Autodesk Inventor part; units mm, degrees
ref_plane "YZ Plane" through (0, 0, 0) normal (1, 0, 0) x (0, 1, 0)
ref_plane "XZ Plane" through (0, 0, 0) normal (0, 1, 0) x (-1, 0, 0)
ref_plane "XY Plane" through (0, 0, 0) normal (0, 0, 1) x (1, 0, 0)
sketch "Sketch1" plane through (0, 0, 0) normal (0, 0, 1) x (1, 0, 0)
  line L0 (0, 0) -> (38.1, 0)
  line L1 (38.1, 0) -> (38.1, 38.1)
  line L2 (38.1, 38.1) -> (0, 38.1)
  line L3 (0, 38.1) -> (0, 0)
  dimension "d0" = 38.1
  dimension "d1" = 38.1
extrude "Extrusion1" add sketch "Sketch1" along normal blind 38.1
sketch "Sketch2" plane through (0, 0, 38.1) normal (0, 0, 1) x (1, 0, 0)
  line L0 (6.35, 6.35) -> (32.004, 6.35)
  line L1 (32.004, 6.35) -> (32.004, 32.004)
  line L2 (32.004, 32.004) -> (6.35, 32.004)
  line L3 (6.35, 32.004) -> (6.35, 6.35)
  line L4 (38.1, 0) -> (38.1, 38.1)
  line L5 (0, 0) -> (38.1, 0)
  line L6 (38.1, 0) -> (38.1, 38.1)
  line L7 (38.1, 38.1) -> (0, 38.1)
  line L8 (0, 38.1) -> (0, 0)
  dimension "d4" = 25.654
  dimension "d5" = 25.654
extrude "Extrusion2" cut sketch "Sketch2" against normal blind 31.75 contours L3 L2 L1 L0
sketch "Sketch5" plane through (0, 0, 38.1) normal (0, 0, 1) x (1, 0, 0)
  line L0 (6.35, 6.35) -> (6.35, 32.004)
  line L1 (6.35, 6.35) -> (32.004, 6.35)
  line L2 (32.004, 6.35) -> (32.004, 32.004)
  line L3 (32.004, 32.004) -> (6.35, 32.004)
  line L4 (6.35, 32.004) -> (6.35, 6.35)
  line L5 (0, 0) -> (38.1, 0)
  line L6 (0, 0) -> (38.1, 0)
  line L7 (38.1, 0) -> (38.1, 38.1)
  line L8 (38.1, 38.1) -> (0, 38.1)
  line L9 (0, 38.1) -> (0, 0)
extrude "Extrusion4" add sketch "Sketch5" along normal blind 38.1
sketch "Sketch7" plane through (38.1, 0, 0) normal (1, 0, 0) x (0, 0, -1)
  line L0 (0, 0) -> (-76.2, 0)
  line L1 (0, 0) -> (-38.1, 0)
  line L2 (-38.1, 0) -> (-38.1, 38.1)
  line L3 (-38.1, 38.1) -> (0, 38.1)
  line L4 (0, 38.1) -> (0, 0)
  line L5 (-76.2, 6.35) -> (-6.35, 6.35)
  line L6 (-6.35, 6.35) -> (-32.004, 6.35)
  line L7 (-32.004, 6.35) -> (-32.004, 32.004)
  line L8 (-32.004, 32.004) -> (-6.35, 32.004)
  line L9 (-6.35, 32.004) -> (-6.35, 6.35)
  dimension "d16" = 38.1
  dimension "d17" = 38.1
  dimension "d20" = 25.654
  dimension "d21" = 25.654
extrude "Extrusion6" add sketch "Sketch7" along normal blind 38.1
sketch "Sketch9" plane through (38.1, 6.35, 6.35) normal (1, 0, 0) x (0, 0, -1)
  line L0 (-25.654, 0) -> (-25.654, 25.654)
  line L1 (0, 0) -> (0, 25.654)
  line L2 (-25.654, 0) -> (0, 0)
  line L3 (0, 0) -> (0, 25.654)
  line L4 (0, 25.654) -> (-25.654, 25.654)
  line L5 (-25.654, 25.654) -> (-25.654, 0)
  point P0 (6.35, -6.35)
extrude "Extrusion7" cut sketch "Sketch9" against normal blind 31.75
sketch "Sketch10" plane through (0, 38.1, 76.2) normal (0, 1, 0) x (1, 0, 0)
  line L0 (76.2, 69.85) -> (6.35, 69.85)
  line L1 (6.35, 69.85) -> (32.004, 69.85)
  line L2 (32.004, 69.85) -> (32.004, 44.196)
  line L3 (32.004, 44.196) -> (6.35, 44.196)
  line L4 (6.35, 44.196) -> (6.35, 69.85)
  line L5 (38.1, 38.1) -> (38.1, 0)
  line L6 (0, 76.2) -> (0, 0)
  line L7 (38.1, 38.1) -> (0, 38.1)
  line L8 (0, 38.1) -> (0, 76.2)
  line L9 (0, 76.2) -> (38.1, 76.2)
  line L10 (38.1, 76.2) -> (38.1, 38.1)
  point P0 (0, 38.1)
  dimension "d26" = 25.654
  dimension "d27" = 25.654
extrude "Extrusion8" add sketch "Sketch10" along normal blind 38.1
sketch "Sketch11" plane through (6.35, 38.1, 6.35) normal (0, 1, 0) x (1, 0, 0)
  line L0 (0, -25.654) -> (25.654, -25.654)
  line L1 (25.654, -25.654) -> (0, -25.654)
  line L2 (0, -25.654) -> (0, 0)
  line L3 (0, 0) -> (25.654, 0)
  line L4 (25.654, 0) -> (25.654, -25.654)
  point P0 (-6.35, 6.35)
extrude "Extrusion9" cut sketch "Sketch11" against normal blind 6.35
sketch "Sketch12" plane through (0, 76.2, 76.2) normal (0, 1, 0) x (1, 0, 0)
  line L0 (38.1, 55.88) -> (32.004, 55.88)
  line L1 (32.004, 55.88) -> (32.004, 58.42)
  line L2 (32.004, 58.42) -> (38.1, 58.42)
  line L3 (38.1, 58.42) -> (38.1, 55.88)
  point P0 (0, 76.2)
  dimension "d32" = 6.096
  dimension "d33" = 2.54
extrude "Extrusion10" cut sketch "Sketch12" against normal blind 38.1
sketch "Sketch13" plane through (76.2, 38.1, 38.1) normal (0, 1, 0) x (1, 0, 0)
  line L0 (0, 31.75) -> (0, 6.096)
  line L1 (-44.196, 17.78) -> (0, 17.78)
  line L2 (0, 17.78) -> (0, 20.32)
  line L3 (0, 20.32) -> (-44.196, 20.32)
  line L4 (-44.196, 20.32) -> (-44.196, 17.78)
  point P0 (-76.2, 38.1)
  dimension "d36" = 2.54
extrude "Extrusion11" cut sketch "Sketch13" against normal blind 6.35
sketch "Sketch15" plane through (0, 76.2, 76.2) normal (0, 1, 0) x (1, 0, 0)
  line L0 (17.78, 38.1) -> (20.32, 38.1)
  line L1 (20.32, 38.1) -> (20.32, 44.196)
  line L2 (20.32, 44.196) -> (17.78, 44.196)
  line L3 (17.78, 44.196) -> (17.78, 38.1)
  point P0 (0, 76.2)
  dimension "d39" = 2.54
  dimension "d40" = 6.096
extrude "Extrusion12" cut sketch "Sketch15" against normal blind 38.1
sketch "Sketch16" plane through (0, 38.1, 76.2) normal (0, 1, 0) x (1, 0, 0)
  line L0 (20.32, 44.196) -> (20.32, 38.1)
  line L1 (0, 0) -> (38.1, 0)
  line L2 (20.32, 44.196) -> (17.78, 44.196)
  line L3 (17.78, 44.196) -> (17.78, 0)
  line L4 (17.78, 0) -> (20.32, 0)
  line L5 (20.32, 0) -> (20.32, 44.196)
  point P0 (0, 76.2)
  dimension "d43" = 2.54
extrude "Extrusion13" cut sketch "Sketch16" against normal blind 6.35
sketch "Sketch17" plane through (38.1, 0, 76.2) normal (1, 0, 0) x (0, 0, -1)
  line L0 (38.1, 0) -> (38.1, 38.1)
  line L1 (0, 17.78) -> (38.1, 17.78)
  line L2 (38.1, 17.78) -> (38.1, 20.32)
  line L3 (38.1, 20.32) -> (0, 20.32)
  line L4 (0, 20.32) -> (0, 17.78)
  point P0 (76.2, 0)
  dimension "d46" = 2.54
extrude "Extrusion14" cut sketch "Sketch17" against normal blind 6.35
sketch "Sketch18" plane through (38.1, 0, 38.1) normal (0, 0, 1) x (1, 0, 0)
  line L0 (0, 17.78) -> (38.1, 17.78)
  line L1 (38.1, 17.78) -> (38.1, 20.32)
  line L2 (38.1, 20.32) -> (0, 20.32)
  line L3 (0, 20.32) -> (0, 17.78)
  point P0 (-38.1, 0)
  dimension "d49" = 38.1
  dimension "d50" = 2.54
extrude "Extrusion15" cut sketch "Sketch18" against normal blind 6.35
sketch "Sketch20" plane through (38.1, 38.1, 38.1) normal (0, 0, 1) x (1, 0, 0)
  line L0 (-17.78, -6.096) -> (-17.78, 38.1)
  line L1 (0, 0) -> (-17.78, 0)
  line L2 (-17.78, 38.1) -> (-16.51, 38.1)
  line L3 (-16.51, 38.1) -> (-16.51, 0)
  line L4 (-16.51, 0) -> (-17.78, 0)
  line L5 (-17.78, 0) -> (-17.78, 38.1)
  point P0 (-38.1, -38.1)
  dimension "d53" = 1.27
extrude "Extrusion16" cut sketch "Sketch20" against normal blind 6.35
sketch "Sketch21" plane through (38.1, 38.1, 76.2) normal (0, 1, 0) x (1, 0, 0)
  line L0 (-17.78, 0) -> (-17.78, 44.196)
  line L1 (0, 0) -> (-17.78, 0)
  line L2 (-17.78, 44.196) -> (-16.51, 44.196)
  line L3 (-16.51, 44.196) -> (-16.51, 0)
  line L4 (-16.51, 0) -> (-17.78, 0)
  line L5 (-17.78, 0) -> (-17.78, 44.196)
  point P0 (-38.1, 76.2)
  dimension "d56" = 1.27
extrude "Extrusion17" cut sketch "Sketch21" against normal blind 6.35
sketch "Sketch23" plane through (0, 38.1, 38.1) normal (0, 0, 1) x (1, 0, 0)
  line L0 (17.78, 0) -> (17.78, 38.1)
  line L1 (17.78, 0) -> (0, 0)
  line L2 (17.78, 38.1) -> (16.51, 38.1)
  line L3 (16.51, 38.1) -> (16.51, 0)
  line L4 (16.51, 0) -> (17.78, 0)
  line L5 (17.78, 0) -> (17.78, 38.1)
  point P0 (0, -38.1)
  dimension "d59" = 1.27
extrude "Extrusion18" cut sketch "Sketch23" against normal blind 6.35
sketch "Sketch24" plane through (0, 38.1, 76.2) normal (0, 1, 0) x (1, 0, 0)
  line L0 (17.78, 44.196) -> (17.78, 0)
  line L1 (17.78, 0) -> (0, 0)
  line L2 (17.78, 44.196) -> (16.51, 44.196)
  line L3 (16.51, 44.196) -> (16.51, 0)
  line L4 (16.51, 0) -> (17.78, 0)
  line L5 (17.78, 0) -> (17.78, 44.196)
  point P0 (0, 76.2)
  dimension "d62" = 1.27
extrude "Extrusion19" cut sketch "Sketch24" against normal blind 6.35
sketch "Sketch25" plane through (38.1, 0, 76.2) normal (1, 0, 0) x (0, 0, -1)
  line L0 (38.1, 0) -> (38.1, 17.78)
  line L1 (38.1, 17.78) -> (0, 17.78)
  line L2 (0, 17.78) -> (0, 16.51)
  line L3 (0, 16.51) -> (38.1, 16.51)
  line L4 (38.1, 16.51) -> (38.1, 17.78)
  point P0 (76.2, 0)
  dimension "d65" = 38.1
  dimension "d66" = 1.27
extrude "Extrusion20" cut sketch "Sketch25" against normal blind 6.35
sketch "Sketch26" plane through (38.1, 38.1, 76.2) normal (1, 0, 0) x (0, 0, -1)
  line L0 (0, -17.78) -> (38.1, -17.78)
  line L1 (38.1, -17.78) -> (0, -17.78)
  line L2 (0, -17.78) -> (0, -16.51)
  line L3 (0, -16.51) -> (38.1, -16.51)
  line L4 (38.1, -16.51) -> (38.1, -17.78)
  point P0 (76.2, -38.1)
  dimension "d69" = 38.1
  dimension "d70" = 1.27
extrude "Extrusion21" cut sketch "Sketch26" against normal blind 6.35
sketch "Sketch27" plane through (38.1, 0, 38.1) normal (0, 0, 1) x (1, 0, 0)
  line L0 (0, 21.59) -> (0, 38.1)
  line L1 (0, 20.32) -> (38.1, 20.32)
  line L2 (0, 21.59) -> (38.1, 21.59)
  line L3 (38.1, 21.59) -> (38.1, 20.32)
  line L4 (38.1, 20.32) -> (0, 20.32)
  line L5 (0, 20.32) -> (0, 21.59)
  line L6 (38.1, 17.78) -> (0, 17.78)
  line L7 (0, 17.78) -> (38.1, 17.78)
  line L8 (38.1, 17.78) -> (38.1, 16.51)
  line L9 (38.1, 16.51) -> (0, 16.51)
  line L10 (0, 16.51) -> (0, 17.78)
  point P0 (-38.1, 0)
  dimension "d73" = 38.1
  dimension "d74" = 1.27
extrude "Extrusion22" cut sketch "Sketch27" against normal blind 6.35
sketch "Sketch28" plane through (38.1, 38.1, 38.1) normal (0, 1, 0) x (1, 0, 0)
  line L0 (0, 20.32) -> (38.1, 20.32)
  line L1 (0, 20.32) -> (38.1, 20.32)
  line L2 (38.1, 20.32) -> (38.1, 21.59)
  line L3 (38.1, 21.59) -> (0, 21.59)
  line L4 (0, 21.59) -> (0, 20.32)
  line L5 (-6.096, 17.78) -> (38.1, 17.78)
  line L6 (38.1, 17.78) -> (0, 17.78)
  line L7 (0, 17.78) -> (0, 16.51)
  line L8 (0, 16.51) -> (38.1, 16.51)
  line L9 (38.1, 16.51) -> (38.1, 17.78)
  point P0 (-38.1, 38.1)
  point P1 (0, 17.78)
  dimension "d77" = 38.1
  dimension "d78" = 1.27
  dimension "d79" = 38.1
  dimension "d80" = 1.27
extrude "Extrusion23" cut sketch "Sketch28" against normal blind 6.35
sketch "Sketch29" plane through (38.1, 38.1, 0) normal (1, 0, 0) x (0, 0, -1)
  line L0 (-17.78, -6.096) -> (-6.35, -6.096)
  line L1 (-6.35, 38.1) -> (-17.78, 38.1)
  line L2 (-17.78, -6.096) -> (-16.51, -6.096)
  line L3 (-16.51, -6.096) -> (-16.51, 38.1)
  line L4 (-16.51, 38.1) -> (-17.78, 38.1)
  line L5 (-17.78, 38.1) -> (-17.78, -6.096)
  line L6 (-21.59, 0) -> (-21.59, -6.096)
  line L7 (-20.32, 38.1) -> (-20.32, -6.096)
  line L8 (-21.59, -6.096) -> (-20.32, -6.096)
  line L9 (-20.32, -6.096) -> (-20.32, 38.1)
  line L10 (-20.32, 38.1) -> (-21.59, 38.1)
  line L11 (-21.59, 38.1) -> (-21.59, -6.096)
  point P0 (0, -38.1)
  point P1 (-20.32, -6.096)
  dimension "d83" = 1.27
extrude "Extrusion24" cut sketch "Sketch29" against normal blind 6.35
sketch "Sketch30" plane through (76.2, 38.1, 21.59) normal (0, 0, -1) x (-1, 0, 0)
  line L0 (0, 0) -> (38.1, 0)
  line L1 (44.196, 38.1) -> (44.196, -6.096)
  line L2 (38.1, 0) -> (44.196, 0)
  line L3 (44.196, 0) -> (44.196, -6.096)
  line L4 (44.196, -6.096) -> (38.1, -6.096)
  line L5 (38.1, -6.096) -> (38.1, 0)
  point P0 (76.2, -38.1)
  point P1 (44.196, 0)
extrude "Extrusion25" add sketch "Sketch30" along normal blind 5.08
sketch "Sketch31" plane through (21.59, 38.1, 38.1) normal (-1, 0, 0) x (0, 0, 1)
  line L0 (38.1, -6.096) -> (-6.096, -6.096)
  line L1 (0, 0) -> (-6.096, 0)
  line L2 (-6.096, 0) -> (-6.096, -6.096)
  line L3 (-6.096, -6.096) -> (0, -6.096)
  line L4 (0, -6.096) -> (0, 0)
  point P0 (-38.1, -38.1)
extrude "Extrusion26" add sketch "Sketch31" along normal blind 5.08
sketch "Sketch32" plane through (0, 0, 76.2) normal (-1, 0, 0) x (0, 0, 1)
  line L0 (0, 38.1) -> (0, 0)
  line L1 (0, 19.05) -> (-76.2, 19.05)
  line L2 (-76.2, 19.05) -> (-76.2, 0)
  line L3 (-76.2, 0) -> (0, 0)
  line L4 (0, 0) -> (0, 19.05)
  line L5 (-76.2, 0) -> (-56.896, 0)
  line L6 (-56.896, 0) -> (-56.896, 76.2)
  line L7 (-56.896, 76.2) -> (-76.2, 76.2)
  line L8 (-76.2, 76.2) -> (-76.2, 0)
  point P0 (0, 0)
  point P1 (-56.896, 19.05)
  dimension "d90" = 19.304
  dimension "d91" = 76.2
extrude "Extrusion27" add sketch "Sketch32" along normal blind 12.7 contours L6 L3 L2 L1 | L1 L8 L7 L6
sketch "Sketch35" plane through (-12.7, 0, 76.2) normal (-1, 0, 0) x (0, 0, 1)
  line L0 (-38.1, 38.1) -> (-38.1, 76.2)
  line L1 (-38.1, 76.2) -> (-56.896, 76.2)
  line L2 (-56.896, 76.2) -> (-56.896, 0)
  line L3 (-56.896, 0) -> (-38.1, 0)
  line L4 (-38.1, 0) -> (-38.1, 76.2)
  point P0 (-76.2, 0)
  dimension "d102" = 18.796
  dimension "d103" = 76.2
extrude "Extrusion30" add sketch "Sketch35" against normal blind 6.35
properties part number "corner connector with rails (front left)"
Build history of the part. All positions in model axes, mm. A direction names the side the tool comes from. Coordinates: 2 decimals unless noted, no trailing zeros. Write each loop counter-clockwise with the first axis right and the second up, starting at its lowest first coordinate (ties: lowest second). Pieces come first, ordered by that corner, then holes. Notation, with made-up numbers: (-21, 49.5) -> (38, 49.5) arc R27 ccw to (38, 80.5) -> close; hole circle Ø8 at (20, 9.25). An arc over 180 degrees is marked (long way). Use CSV: the item, a comma, the result in double quotes. Start each with the question number.
Q1. Cut at A-A, the plane z = 23.5. List the corners of the cut face in (x, y), then the cut area to 3 significant figures.
Q2. Cut at C-C, the plane y = 23. List the corners of the cut face in (x, z).
Q3. 3-axis set-ups, long thin cutter, end or side, ignore diameter. For faces 1 (the flat face through (57, 30, 38.1)), 2 (the flat face through (21.59, 57, 35)), 3 (the flat face through (57, 35, 21.59)): which of +Z, -Z, +X, -X, +Y, -Y reach the whole face in a straight line?
Q4. Cut at D-D, the plane z = 61. List the corners of the cut face in (x, y).
Q5. Pull direction Z, two halves, no side cores. Call faces 4 (the flat face through (-6.35, 39, 29)), 5 (the flat face through (38.1, 35, 19)), 6 (the flat face through (-3, 38, 19.304)): released by +Z, released by -Z, zero draft, split by the parting line, or undercut.
Q6. Cut at B-B, the plane x = 11.5. List the corners of the cut face in (y, z), then the cut area to 3 significant figures.
Q7. Drill centre lines: probe 1 along X at (y, z) = (59.5, 30.5); probe 2 along X at (y, z) = (37.5, 70.5); probe 3 along Z at (x, y) = (44, 25.5). Where is each one in solid material? Low to high.
Q8. Flat gauge pins, fed straight in: pin 1 Ø6.5 at (x, y) = (57, 36.5) entering from +Z; pin 2 Ø1.5 at (x, z) = (1, 52.5) entering from +Y; pin 3 Ø5 at (y, z) = (19.5, 48) entering from -X. Where does each tip first touch, or does it go through?
Checked values:
1,outline,"(-12.7, 0) -> (-6.35, 0) -> (-6.35, 76.2) -> (-12.7, 76.2) -> close; (0, 0) -> (76.2, 0) -> (76.2, 6.35) -> (6.35, 6.35) -> (6.35, 76.2) -> (0, 76.2) -> close; (32, 32) -> (76.2, 32) -> (76.2, 38.1) -> (38.1, 38.1) -> (38.1, 76.2) -> (32, 76.2) -> close"
1,area,"1,910 mm²"
2,outline,"(-12.7, 0) -> (76.2, 0) -> (76.2, 6.35) -> (6.35, 6.35) -> (6.35, 76.2) -> (0, 76.2) -> (0, 19.3) -> (-6.35, 19.3) -> (-6.35, 38.1) -> (-12.7, 38.1) -> close; (32, 32) -> (76.2, 32) -> (76.2, 38.1) -> (38.1, 38.1) -> (38.1, 76.2) -> (32, 76.2) -> close"
3,face 1,"+Z, +X, +Y, -Y"
3,face 2,"+Z, +Y"
3,face 3,"+X, +Y"
4,outline,"(0, 0) -> (38.1, 0) -> (38.1, 16.51) -> (32, 16.51) -> (32, 6.35) -> (6.35, 6.35) -> (6.35, 32) -> (16.51, 32) -> (16.51, 38.1) -> (0, 38.1) -> close; (21.59, 32) -> (32, 32) -> (32, 21.59) -> (38.1, 21.59) -> (38.1, 38.1) -> (21.59, 38.1) -> close"
5,face 4,"zero draft"
5,face 5,"undercut"
5,face 6,"released by +Z"
6,outline,"(0, 0) -> (76.2, 0) -> (76.2, 6.35) -> (6.35, 6.35) -> (6.35, 76.2) -> (0, 76.2) -> close; (32, 32) -> (76.2, 32) -> (76.2, 38.1) -> (38.1, 38.1) -> (38.1, 76.2) -> (32, 76.2) -> close"
6,area,"1,430 mm²"
7,probe 1,"x = -12.7 to -6.35, 0 to 6.35, 32 to 38.1"
7,probe 2,"x = 0 to 16.51, 21.59 to 38.1"
7,probe 3,"z = 0 to 6.35, 32 to 38.1"
8,pin 1,"stops at z = 38.1"
8,pin 2,"stops at y = 38.1"
8,pin 3,"stops at x = 0"
